Model file for the job. Use its own axes, mm. Face numbers are marked on the shaded views. A direction names the side the tool comes from. Coordinates: 2 decimals unless noted, no trailing zeros. Loops run counter-clockwise (first coordinate to the right, second up) from the corner with the lowest first, then second, coordinate; pieces in that order, holes last. Notation, with made-up numbers: M 44,26.25 L 51,26.25 A29 cw 51,65.25 Z; hole C 85,13 d6. An arc over 180 degrees is marked long. One line per question, with ' | ' between items. Start each with the question number.
```python
from build123d import *

# Parameters (mm, degrees)
SKETCH1_R             = 12.5
BOSS_EXTRUDE1_DEPTH   = 4.4
SKETCH2_R             = 10.95
BOSS_EXTRUDE2_DEPTH   = 1
SKETCH3_R             = 10.05
CUT_EXTRUDE1_DEPTH    = 3
SKETCH4_R             = 3.5
CUT_EXTRUDE2_DEPTH    = 18.930421077
SKETCH5_R             = 1.4
CUT_EXTRUDE3_DEPTH    = 19.484047176
SKETCH6_R             = 1.4
BOSS_EXTRUDE3_DEPTH   = 3
FILLET1_R             = 0.5
SKETCH7_R             = 2.5
CUT_EXTRUDE4_DEPTH    = 2.65
M3X0_5_TAPPED_HOLE1_D = 2.5


with BuildPart() as part:
    # Sketch1 → Boss-Extrude1 (new body)
    with BuildSketch(Plane(origin=(0, 0, 0), x_dir=(1, 0, 0), z_dir=(0, 1, 0))):
        with Locations(Location((0, 0, 0), (0, 0, 270))):
            Circle(SKETCH1_R)
    extrude(amount=BOSS_EXTRUDE1_DEPTH)

    # Sketch2 → Boss-Extrude2 (add)
    with BuildSketch(Plane(origin=(0, 4.4, 0), x_dir=(1, 0, 0), z_dir=(0, 1, 0))):
        with Locations(Location((0, 0, 0), (0, 0, 270))):
            Circle(SKETCH2_R)
    extrude(amount=BOSS_EXTRUDE2_DEPTH)

    # Sketch3 → Cut-Extrude1 (cut)
    with BuildSketch(Plane(origin=(0, 5.4, 0), x_dir=(1, 0, 0), z_dir=(0, 1, 0))):
        with Locations(Location((0, 0, 0), (0, 0, 270))):
            Circle(SKETCH3_R)
    extrude(amount=-CUT_EXTRUDE1_DEPTH, mode=Mode.SUBTRACT)

    # Sketch4 → Cut-Extrude2 (cut, through all)
    with BuildSketch(Plane(origin=(0, 2.4, 0), x_dir=(1, 0, 0), z_dir=(0, 1, 0))):
        with Locations(Location((0, 0, 0), (0, 0, 270))):
            Circle(SKETCH4_R)
    extrude(amount=-CUT_EXTRUDE2_DEPTH, mode=Mode.SUBTRACT)

    # Sketch5 → Cut-Extrude3 (cut, through all)
    with BuildSketch(Plane.XZ):
        with Locations(Location((-8.5, 0, 0), (0, 0, 270))):
            Circle(SKETCH5_R)
        with Locations(Location((8.5, 0, 0), (0, 0, 270))):
            Circle(SKETCH5_R)
    extrude(amount=-CUT_EXTRUDE3_DEPTH, mode=Mode.SUBTRACT)

    # Sketch6 → Boss-Extrude3 (add)
    # profile 1 of 2: a face of its own
    with BuildSketch(Plane(origin=(0, 2.4, 0), x_dir=(1, 0, 0), z_dir=(0, 1, 0))):
        with BuildLine():
            ThreePointArc((-9.696617647, 2.641610533), (-5.6, 0), (-9.696617647, -2.641610533))
            ThreePointArc((-9.696617647, -2.641610533), (-10.05, 0), (-9.696617647, 2.641610533))
        make_face()
        with Locations(Location((-8.5, 0, 0), (0, 0, 90))):
            Circle(SKETCH6_R, mode=Mode.SUBTRACT)
    # profile 2 of 2: a face of its own
    with BuildSketch(Plane(origin=(0, 2.4, 0), x_dir=(1, 0, 0), z_dir=(0, 1, 0))):
        with BuildLine():
            ThreePointArc((9.696617647, -2.641610533), (5.6, 0), (9.696617647, 2.641610533))
            ThreePointArc((9.696617647, 2.641610533), (10.05, 0), (9.696617647, -2.641610533))
        make_face()
        with Locations(Location((8.5, 0, 0), (0, 0, 90))):
            Circle(SKETCH6_R, mode=Mode.SUBTRACT)
    extrude(amount=BOSS_EXTRUDE3_DEPTH)

    # Fillet1
    # the kernel refuses this fillet: 0.5 mm, written as the material it adds along each edge
    with BuildSketch(Plane(origin=(-9.696617647, 0.016337815, 2.641610533), x_dir=(0.30831902274011397, 0, 0.9512830179376593), z_dir=(0, 1, 0)), Plane(origin=(9.696617647, 0.016337815, -2.641610533), x_dir=(-0.30831902274011413, 0, -0.9512830179376593), z_dir=(0, 1, 0))) as fillet1_piece_1:
        with BuildLine():
            CenterArc((0.929746842, 0.499437138), FILLET1_R, 154.693905627, 118.025000924)
            ThreePointArc((0.477728298, 0.713164151), (0.265396902, 0.338808542), (0, 0))
            ThreePointArc((0, 0), (0.476732437, -0.011313523), (0.953464874, 0))
        make_face()
    extrude(amount=5.383662185)
    with BuildSketch(Plane(origin=(-9.696617647, 0.016337815, -2.641610533), x_dir=(0.9619368896352812, 0, -0.2732716969589074), z_dir=(0, 1, 0)), Plane(origin=(9.696617647, 0.016337815, 2.641610533), x_dir=(-0.9619368896352809, 0, 0.2732716969589082), z_dir=(0, 1, 0))) as fillet1_piece_2:
        with BuildLine():
            CenterArc((0.932385368, 0.494493854), FILLET1_R, 143.464092257, 118.025000924)
            ThreePointArc((0.530643407, 0.792157081), (0.255922209, 0.402374993), (0, 0))
            ThreePointArc((0, 0), (0.429193265, 0.031935645), (0.858386529, 0))
        make_face()
    extrude(amount=5.383662185)

    # Sketch7 → Cut-Extrude4 (cut)
    with BuildSketch(Plane.XZ):
        with Locations(Location((-8.5, 0, 0), (0, 0, 270))):
            Circle(SKETCH7_R)
        with Locations(Location((8.5, 0, 0), (0, 0, 270))):
            Circle(SKETCH7_R)
    extrude(amount=-CUT_EXTRUDE4_DEPTH, mode=Mode.SUBTRACT)

    # M3x0.5 Tapped Hole1 (through all)
    with Locations(Plane(origin=(0, 0, 0), x_dir=(-1, 0, 0), z_dir=(0, -1, 0))):
        with Locations((0, 8.5), (0, -8.5)):
            Hole(M3X0_5_TAPPED_HOLE1_D / 2)


solid = part.part
```
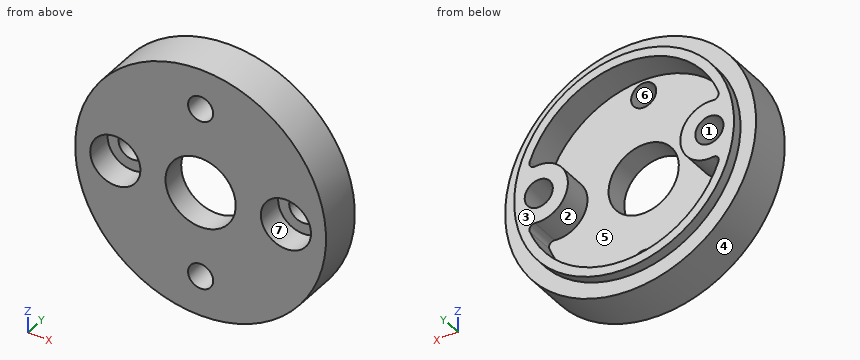
(1) Band-saw the part on D-D on z = -8.5. Write the cut outline in (x, y), then the cut area to 3 significant figures.
(2) Band-saw the part on B-B on z = 0. Give the number of separate pieces and of enclosed holes in the cut face, then the cut area to 3 significant figures.
(3) Drill centre lines: line 1 (X direction, y = 1.8, z = 0); line 2 (X direction, y = 5.05, z = -0.5); line 3 (Y direction, x = -9.25, z = 2). Where is each one in solid material? Low to high. Write a range as [from, to].
(4) Two-plate mould, pull along X, no slides. Class the marked faces 1, 2, 3 and 4: pulls with the +X half, pulls with the -X half, needs draft (parallel to the pull), parting line crosses it, or undercut.
(5) Band-saw the part on A-A on x = 0. Write the cut outline in (y, z).
(6) 3-axis set-ups, long thin cutter, end or side, ignore diameter. For the marked faces 5, 6 and 7: which of +Z, -Z, +X, -X, +Y, -Y reach the whole face in a straight line?
(7) Pin check, flat tips, straight feed: P1, Ø2, axis at y = 4, z = 6, coming from the +X side; P2, Ø9, axis at x = 0, z = 0, coming from the +Y side; P3, Ø1, axis at x = 7.5, y = 4, coming from the -Z side; P4, Ø15, axis at x = 4, z = 4, coming from the +Y side. Stop position of each tip, or through.
(8) Band-saw the part on C-C on x = -8. Write the cut outline in (y, z), then the cut area to 3 significant figures.
Computed values:
1) outline: M -9.17,0 L -1.25,0 L -1.25,2.4 L -5.36,2.4 L -5.36,5.4 L -6.9,5.4 L -6.9,4.4 L -9.17,4.4 Z; M 1.25,0 L 9.17,0 L 9.17,4.4 L 6.9,4.4 L 6.9,5.4 L 5.36,5.4 L 5.36,2.4 L 1.25,2.4 Z | area: 56.3 mm^2
2) separate pieces: 4 | enclosed holes: 0 | area: 39.6 mm^2
3) line 1: [-12.5, -11], [-6, -3.5], [3.5, 6], [11, 12.5] | line 2: [-10.94, -9.81], [-7.19, -5.64], [5.64, 7.19], [9.81, 10.94] | line 3: [2.65, 5.4]
4) face 1: undercut | face 2: undercut | face 3: needs draft | face 4: parting line crosses it
5) outline: M 0,-12.5 L 4.4,-12.5 L 4.4,-10.95 L 5.4,-10.95 L 5.4,-10.05 L 2.4,-10.05 L 2.4,-9.75 L 0,-9.75 Z; M 0,-7.25 L 2.4,-7.25 L 2.4,-3.5 L 0,-3.5 Z; M 0,3.5 L 2.4,3.5 L 2.4,7.25 L 0,7.25 Z; M 0,9.75 L 2.4,9.75 L 2.4,10.05 L 5.4,10.05 L 5.4,10.95 L 4.4,10.95 L 4.4,12.5 L 0,12.5 Z
6) face 5: +Y | face 6: +Y, -Y | face 7: -Y
7) P1: x = 11.46 | P2: y = 2.4 | P3: z = -10.36 | P4: y = 5.4
8) outline: M 0,-9.6 L 4.4,-9.6 L 4.4,-7.48 L 5.4,-7.48 L 5.4,-6.08 L 2.4,-6.08 L 2.4,-2.86 L 5.4,-2.86 L 5.4,-1.31 L 2.65,-1.31 L 2.65,-2.45 L 0,-2.45 Z; M 0,2.45 L 2.65,2.45 L 2.65,1.31 L 5.4,1.31 L 5.4,2.86 L 2.4,2.86 L 2.4,6.08 L 5.4,6.08 L 5.4,7.48 L 4.4,7.48 L 4.4,9.6 L 0,9.6 Z | area: 59.9 mm^2
